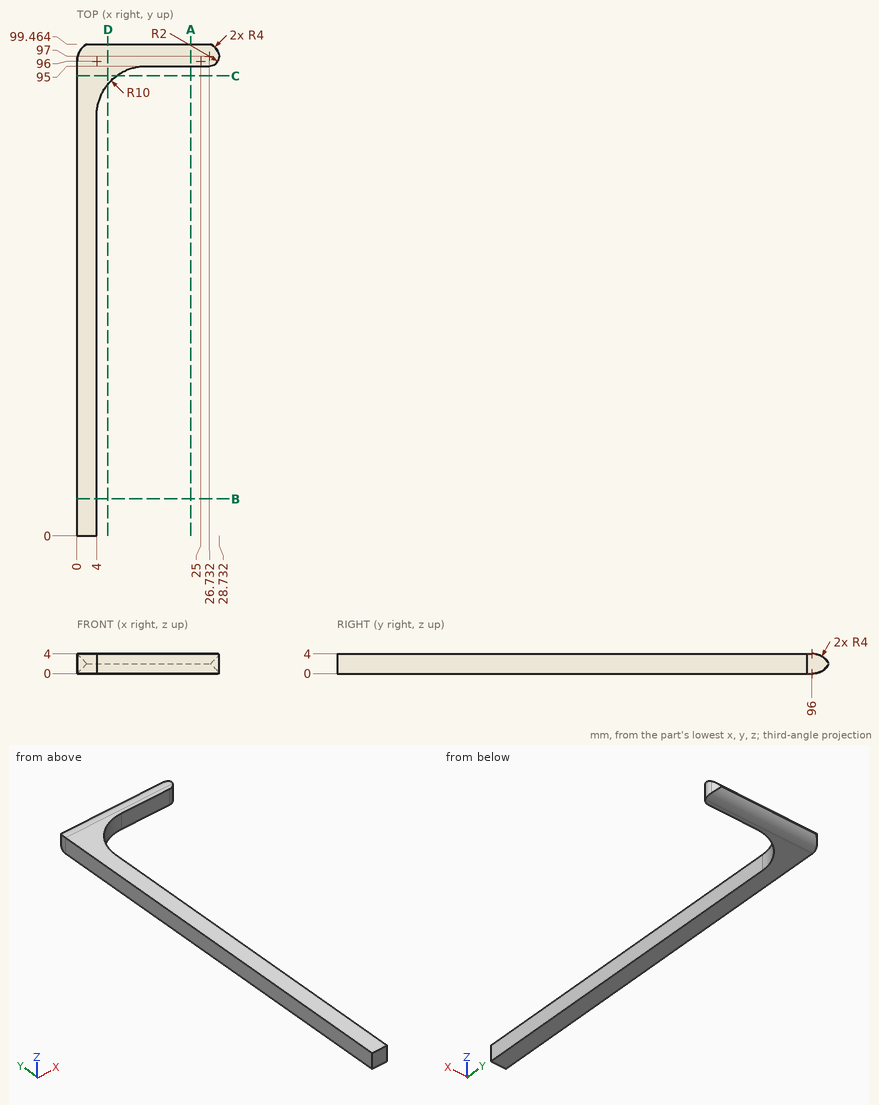
Source: three-view drawing plus pictorial views. Frame: mm from the lowest corner of the part. Round coordinates to 2 decimals unless told otherwise and drop trailing zeros. Write each loop counter-clockwise with the first axis right and the second up, starting at its lowest first coordinate (ties: lowest second). Pieces come first, ordered by that corner, then holes. Notation, with made-up numbers: M 80,47 L 123,47 A20 cw 123,76 Z; hole C -3.5,-18 d11. An arc over 180 degrees is marked long. Use CSV: the item, a comma, the result in double quotes. Start each with the question number.
Q1. Line query: line 1 (X direction, y = 69.5, z = 2.55); line 2 (X direction, y = 94, z = 0.25); line 3 (Y direction, x = 2, z = 2.2). Output: solid intervals per line, ascending. Write a range as from..to.
Q2. Cut plane A-A on x = 23. Output: boundary loops of the cut face in (y, z), plus the area to 3 significant figures.
Q3. Cut plane C-C on y = 93. Output: boundary loops of the cut face in (x, z), plus the area to 3 significant figures.
Q4. First-contact query: P1, Ø2, axis at x = 24.5, z = 3, coming from the -Y side; P2, Ø1.5, axis at y = 56, z = 2, coming from the +X side. Flat tips, straight axial feed; report the tip coordinate or a pass-through.
Q5. Cut plane B-B on y = 7.5. Output: boundary loops of the cut face in (x, z).
Q6. Cut plane D-D on x = 6.25. Output: boundary loops of the cut face in (y, z).
Results found:
1,line 1,"0..4"
1,line 2,"0..9.64"
1,line 3,"0..99.34"
2,outline,"M 95,0 L 96,0 A4 ccw 99.46,2 A4 ccw 96,4 L 95,4 Z"
2,area,"13.8 mm^2"
3,outline,"M 0,0 L 8,0 L 8,4 L 0,4 Z"
3,area,"32.0 mm^2"
4,P1,"y = 95"
4,P2,"x = 4"
5,outline,"M 0,0 L 4,0 L 4,4 L 0,4 Z"
6,outline,"M 91.32,0 L 96,0 A4 ccw 99.46,2 A4 ccw 96,4 L 91.32,4 Z"
